Model file for the job. Use its own axes, mm. A direction names the side the tool comes from. Give positions to 0.01 mm unless a question says otherwise; leave off trailing zeros. Loops run counter-clockwise (first coordinate to the right, second up) from the corner with the lowest first, then second, coordinate; pieces in that order, holes last. Notation, with made-up numbers: (20, 41.5) -> (68, 41.5) arc R24 ccw to (68, 69.5) -> close; hole circle Ø1 at (25, -12.5). An arc over 180 degrees is marked (long way). Use CSV: the item, a comma, the result in double quotes. Start each with the question number.
(1) Drill centre lines: probe 1 along Y at (x, z) = (-5.5, 12.5); probe 2 along X at (y, z) = (-26.4, 25). Where is each one in solid material? Low to high.
(2) 3-axis set-ups, long thin cutter, end or side, ignore diameter. For faces 1 (the cylindrical face through (-27, 0, -22)), 2 (the flat face through (-11.25, -27, 7)), 3 (the flat face through (11.25, 27, 8)), 4 (the flat face through (0, -26, 19)): which of +Z, -Z, +X, -X, +Y, -Y reach the whole face in a straight line?
(3) Flat gauge pins, fed straight in: pin 1 (4 mm diameter, centred on x = -3, y = -10.5, fed in from -Z); pin 2 (10 mm diameter, centred on x = -21, y = -1.5, fed in from +Z); pin 3 (10 mm diameter, centred on x = -21.5, z = -11, fed in from -Y); pin 4 (5 mm diameter, centred on y = 0, z = -23.5, fed in from +X). Where does each tip first touch, or does it go through?
(4) Cut at D-D on y = -8.5. Write the cut outline in (x, z), then the cut area to 3 significant figures.
(5) Pull direction X, two halves, no side cores. Call faces 5 (the flat face through (-27, 11.25, -5)), 6 (the cylindrical face through (-8.4, 26.76, 31.99)), 7 (the cylindrical face through (-25.43, -0.16, -0.6)), 8 (the cylindrical face through (0.07, -26.74, 23.5)): pulls with the +X half, pulls with the -X half, needs draft (parallel to the pull), parting line crosses it, or undercut.
(6) Cut at C-C on z = 16. Write the cut outline in (x, y).
(7) Cut at A-A on x = 0. Write the cut outline in (y, z), then the cut area to 3 significant figures.
(8) Cut at B-B on y = 0. Write the cut outline in (x, z).
from build123d import *

# Parameters (mm, degrees)
EXTRUDE_1_DEPTH     = 11.25
SKETCH_2_R          = 1.5
CUT_EXTRUDE_1_DEPTH = 67.155593112
SKETCH_3_W          = 55
SKETCH_3_H          = 22.5
EXTRUDE_1_2_DEPTH   = 1.5
SKETCH_4_W          = 1.5
SKETCH_4_H          = 22.5
EXTRUDE_2_DEPTH     = 35
SKETCH_5_R          = 1.5
CUT_EXTRUDE_2_DEPTH = 71.75485849
FILLET_1_R          = 10
FILLET_2_R          = 2


with BuildPart() as part:
    # 草图1 → Extrude 1 (new, symmetric)
    with BuildSketch(Plane(origin=(0, 0, 0), x_dir=(0, 0, -1), z_dir=(1, 0, 0))):
        Polygon((-35, 27.5), (0, 27.5), (0, -27.5), (-35, -27.5), (-35, -26), (-1.5, -26), (-1.5, 26), (-35, 26), align=None)
    extrude(amount=EXTRUDE_1_DEPTH, both=True)

    # 草图2 → 切除-拉伸1 (cut, through all)
    with BuildSketch(Plane(origin=(0, 27.5, 0), x_dir=(1, 0, 0), z_dir=(0, 1, 0))):
        with Locations(Location((0, -25, 0), (0, 0, 270))):
            Circle(SKETCH_2_R)
    extrude(amount=-CUT_EXTRUDE_1_DEPTH, mode=Mode.SUBTRACT)

    # 草图3 → Extrude 1 2 (add)
    with BuildSketch(Plane(origin=(0, 0, 0), x_dir=(-1, 0, 0), z_dir=(0, 0, -1))):
        Rectangle(SKETCH_3_W, SKETCH_3_H)
    extrude(amount=-EXTRUDE_1_2_DEPTH)

    # 草图4 → 凸台-拉伸2 (add)
    with BuildSketch(Plane.XY.offset(1.5)):
        with Locations((26.75, 0)):
            Rectangle(SKETCH_4_W, SKETCH_4_H)
    extrude_2 = extrude(amount=-EXTRUDE_2_DEPTH)

    # 镜向1: 凸台-拉伸2 across plane
    add(extrude_2.mirror(Plane(origin=(0, 0, 0), x_dir=(0, 0, 1), z_dir=(1, 0, 0))))

    # 草图5 → 切除-拉伸2 (cut, through all)
    with BuildSketch(Plane(origin=(27.5, 0, 0), x_dir=(0, 0, -1), z_dir=(1, 0, 0))):
        with Locations((23.5, 0)):
            Circle(SKETCH_5_R)
    extrude(amount=-CUT_EXTRUDE_2_DEPTH, mode=Mode.SUBTRACT)

    # 圆角1
    fillet_1_edges = [part.edges().sort_by_distance(p)[0] for p in [
        (11.25, 26.75, 35),
        (11.25, -26.75, 35),
        (-11.25, 26.75, 35),
        (26.75, 11.25, -33.5),
        (26.75, -11.25, -33.5),
        (-11.25, -26.75, 35),
        (-26.75, -11.25, -33.5),
        (-26.75, 11.25, -33.5),
    ]]
    fillet(fillet_1_edges, radius=FILLET_1_R)

    # 圆角2
    fillet_2_edges = [part.edges().sort_by_distance(p)[0] for p in [
        (0, -26, 1.5),
        (0, 26, 1.5),
        (0, 27.5, 0),
        (0, -27.5, 0),
        (27.5, 0, 1.5),
        (-27.5, 0, 1.5),
        (26, 0, 0),
        (-26, 0, 0),
    ]]
    fillet(fillet_2_edges, radius=FILLET_2_R)


solid = part.part
Check result:
1,probe 1,"-27.5 to -26, 26 to 27.5"
1,probe 2,"-11.25 to -1.5, 1.5 to 11.25"
2,face 1,"+X, -X"
2,face 2,"+Z, -Z, -X, -Y"
2,face 3,"+Z, -Z, +X, +Y"
2,face 4,"+Z, +X, -X"
3,pin 1,"z = 0"
3,pin 2,"z = 1.5"
3,pin 3,"y = -11.25"
3,pin 4,"x = 27.5"
4,outline,"(-27.5, -30.39) -> (-26, -30.39) -> (-26, -2) arc R2 cw to (-24, 0) -> (24, 0) arc R2 cw to (26, -2) -> (26, -30.39) -> (27.5, -30.39) -> (27.5, -0.5) arc R2 ccw to (25.5, 1.5) -> (-25.5, 1.5) arc R2 ccw to (-27.5, -0.5) -> close"
4,area,"174 mm²"
5,face 5,"needs draft"
5,face 6,"pulls with the -X half"
5,face 7,"undercut"
5,face 8,"undercut"
6,outline,"(-11.25, -27.5) -> (11.25, -27.5) -> (11.25, -26) -> (-11.25, -26) -> close; (-11.25, 26) -> (11.25, 26) -> (11.25, 27.5) -> (-11.25, 27.5) -> close"
7,outline,"(-27.5, 2) arc R2 ccw to (-25.5, 0) -> (25.5, 0) arc R2 ccw to (27.5, 2) -> (27.5, 23.5) -> (26, 23.5) -> (26, 3.5) arc R2 cw to (24, 1.5) -> (-24, 1.5) arc R2 cw to (-26, 3.5) -> (-26, 23.5) -> (-27.5, 23.5) -> close; (-27.5, 26.5) -> (-26, 26.5) -> (-26, 35) -> (-27.5, 35) -> close; (26, 26.5) -> (27.5, 26.5) -> (27.5, 35) -> (26, 35) -> close"
7,area,"174 mm²"
8,outline,"(-27.5, -33.5) -> (-26, -33.5) -> (-26, -25) -> (-27.5, -25) -> close; (-27.5, -22) -> (-26, -22) -> (-26, -2) arc R2 cw to (-24, 0) -> (24, 0) arc R2 cw to (26, -2) -> (26, -22) -> (27.5, -22) -> (27.5, -0.5) arc R2 ccw to (25.5, 1.5) -> (-25.5, 1.5) arc R2 ccw to (-27.5, -0.5) -> close; (26, -33.5) -> (27.5, -33.5) -> (27.5, -25) -> (26, -25) -> close"
